Build history of the part. All positions in model axes, mm. Round coordinates to 2 decimals unless told otherwise and drop trailing zeros. Write each loop counter-clockwise with the first axis right and the second up, starting at its lowest first coordinate (ties: lowest second). Pieces come first, ordered by that corner, then holes. Notation, with made-up numbers: M 46,81.25 L 73,81.25 A25 cw 73,120.25 Z; hole C -2.75,15 d9. An arc over 180 degrees is marked long. Use a Markdown table: item, result.
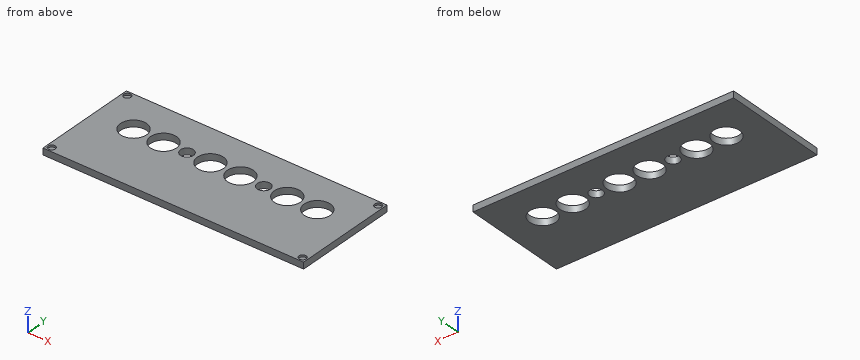
from build123d import *

# Parameters (mm, degrees)
CROQUIS1_W              = 200
CROQUIS1_H              = 80
SALIENTE_EXTRUIR1_DEPTH = 5
CROQUIS2_R              = 2.75
CORTAR_EXTRUIR1_DEPTH   = 1.5
CROQUIS4_R              = 10
CROQUIS4_R_2            = 5
CORTAR_EXTRUIR3_DEPTH   = 5


with BuildPart() as part:
    # Croquis1 → Saliente-Extruir1 (new body)
    with BuildSketch(Plane.XY):
        Rectangle(CROQUIS1_W, CROQUIS1_H)
    extrude(amount=SALIENTE_EXTRUIR1_DEPTH)

    # Croquis2 → Cortar-Extruir1 (cut)
    with BuildSketch(Plane.XY.offset(5)):
        with Locations((-96.25, 36.25)):
            Circle(CROQUIS2_R)
        with Locations((96.25, 36.25)):
            Circle(CROQUIS2_R)
        with Locations((96.25, -36.25)):
            Circle(CROQUIS2_R)
        with Locations((-96.25, -36.25)):
            Circle(CROQUIS2_R)
    extrude(amount=-CORTAR_EXTRUIR1_DEPTH, mode=Mode.SUBTRACT)

    # Croquis4 → Cortar-Extruir3 (cut)
    with BuildSketch(Plane.XY.offset(5)):
        with Locations((-70.5, 10)):
            Circle(CROQUIS4_R)
        with Locations((-47.5, 10)):
            Circle(CROQUIS4_R)
        with Locations((-29.5, 10)):
            Circle(CROQUIS4_R_2)
        with Locations((-11.5, 10)):
            Circle(CROQUIS4_R)
        with Locations((11.5, 10)):
            Circle(CROQUIS4_R)
        with Locations((29.5, 10)):
            Circle(CROQUIS4_R_2)
        with Locations((47.5, 10)):
            Circle(CROQUIS4_R)
        with Locations((70.5, 10)):
            Circle(CROQUIS4_R)
    extrude(amount=-CORTAR_EXTRUIR3_DEPTH, mode=Mode.SUBTRACT)


solid = part.part
Q1. Cut at B-B on z = 4.25. Count the separate pieces of the cut face and the enclosed holes in it, and give its area (3 significant figures).
Response values:
| item | result |
|---|---|
| separate pieces | 1 |
| enclosed holes | 12 |
| area | 13,900 mm2 |
Q2. Drill centre lines: L1, parallel to Y at x = 96.25, z = 4; L2, parallel to Y at x = -11.5, z = 3.2; L3, parallel to Y at x = -28, z = 4.55. Where is each one in solid material? Low to high.
Response values:
| item | result |
|---|---|
| L1 | y = -40 to -39, -33.5 to 33.5, 39 to 40 |
| L2 | y = -40 to 0, 20 to 40 |
| L3 | y = -40 to 5.23, 14.77 to 40 |
Q3. Cut at A-A on x = 47.5. Give the cut face in (y, z), and give its area (3 significant figures).
Response values:
| item | result |
|---|---|
| outline | M -40,0 L 0,0 L 0,5 L -40,5 Z; M 20,0 L 40,0 L 40,5 L 20,5 Z |
| area | 300 mm2 |
Q4. Cut at D-D on x = 96.25. Give the cut face in (y, z), and give its area (4 significant figures).
Response values:
| item | result |
|---|---|
| outline | M -40,0 L 40,0 L 40,5 L 39,5 L 39,3.5 L 33.5,3.5 L 33.5,5 L -33.5,5 L -33.5,3.5 L -39,3.5 L -39,5 L -40,5 Z |
| area | 383.5 mm2 |
Q5. Drop a flat-ended pin along its axis: P1, Ø3, axis at x = 97, y = 37, coming from the +Z side. Give the stop position or say it passes through.
Response values:
| item | result |
|---|---|
| P1 | stops at z = 3.5 |
Q6. Cut at C-C on y = -36.25. Give the cut face in (x, z).
Response values:
| item | result |
|---|---|
| outline | M -100,0 L 100,0 L 100,5 L 99,5 L 99,3.5 L 93.5,3.5 L 93.5,5 L -93.5,5 L -93.5,3.5 L -99,3.5 L -99,5 L -100,5 Z |
